```python
from build123d import *

# Parameters (mm, degrees)
SKETCH1_R           = 150
BOSS_EXTRUDE1_DEPTH = 10
SKETCH2_R           = 2
CUT_EXTRUDE1_DEPTH  = 10


with BuildPart() as part:
    # Sketch1 → Boss-Extrude1 (new body)
    with BuildSketch(Plane(origin=(0, 0, 0), x_dir=(1, 0, 0), z_dir=(0, 1, 0))):
        with Locations(Location((0, 0, 0), (0, 0, 270))):
            Circle(SKETCH1_R)
    extrude(amount=BOSS_EXTRUDE1_DEPTH)

    # Sketch2 → Cut-Extrude1 (cut)
    with BuildSketch(Plane(origin=(0, 10, 0), x_dir=(1, 0, 0), z_dir=(0, 1, 0))):
        with Locations(Location((-14.945, 131.706442493, 0), (0, 0, 270))):
            Circle(SKETCH2_R)
        with Locations(Location((-14.945, 107.646442493, 0), (0, 0, 270))):
            Circle(SKETCH2_R)
        with Locations(Location((14.945, 107.646442493, 0), (0, 0, 90))):
            Circle(SKETCH2_R)
        with Locations(Location((14.945, 131.706442493, 0), (0, 0, 90))):
            Circle(SKETCH2_R)
        with Locations(Location((131.706442493, 14.945, 0), (0, 0, 270))):
            Circle(SKETCH2_R)
        with Locations(Location((131.706442493, -14.945, 0), (0, 0, 90))):
            Circle(SKETCH2_R)
        with Locations(Location((107.646442493, -14.945, 0), (0, 0, 90))):
            Circle(SKETCH2_R)
        with Locations(Location((107.646442493, 14.945, 0), (0, 0, 270))):
            Circle(SKETCH2_R)
        with Locations(Location((14.945, -131.706442493, 0), (0, 0, 270))):
            Circle(SKETCH2_R)
        with Locations(Location((-14.945, -131.706442493, 0), (0, 0, 90))):
            Circle(SKETCH2_R)
        with Locations(Location((-14.945, -107.646442493, 0), (0, 0, 90))):
            Circle(SKETCH2_R)
        with Locations(Location((14.945, -107.646442493, 0), (0, 0, 270))):
            Circle(SKETCH2_R)
        with Locations(Location((-131.706442493, -14.945, 0), (0, 0, 270))):
            Circle(SKETCH2_R)
        with Locations(Location((-131.706442493, 14.945, 0), (0, 0, 90))):
            Circle(SKETCH2_R)
        with Locations(Location((-107.646442493, 14.945, 0), (0, 0, 90))):
            Circle(SKETCH2_R)
        with Locations(Location((-107.646442493, -14.945, 0), (0, 0, 270))):
            Circle(SKETCH2_R)
    extrude(amount=-CUT_EXTRUDE1_DEPTH, mode=Mode.SUBTRACT)


solid = part.part
```
Here's how the part is built. I have some questions about the finished solid (model axes, mm). Coordinates: 2 decimals unless noted, no trailing zeros. Loops run counter-clockwise (first coordinate to the right, second up) from the corner with the lowest first, then second, coordinate; pieces in that order, holes last. Notation, with made-up numbers: M 51,-26.5 L 68,-26.5 A25 ccw 68,-2.5 Z; hole C 72.5,-17.5 d3. An arc over 180 degrees is marked long. One line per item, written item: value.
1. Imagine slicing it at C-C (z = 50.5). List the corners of the cut face in (x, y) for me.
Geometry says:
outline: M -141.24,0 L 141.24,0 L 141.24,10 L -141.24,10 Z
2. Imagine slicing it at A-A (y = 2). State how many separate pieces and enclosed holes the cut face has, and give its area (3 significant figures).
Geometry says:
separate pieces: 1
enclosed holes: 16
area: 70,500 mm2
3. Please list where these lines run through material, in increasing order: probe 1 along Z at (x, y) = (106.5, 5); probe 2 along Z at (x, y) = (16.5, 9); probe 3 along X at (y, z) = (9.25, -132.5).
Geometry says:
probe 1: z = -105.63 to -16.58, -13.31 to 13.31, 16.58 to 105.63
probe 2: z = -149.09 to -132.96, -130.45 to -108.9, -106.39 to 106.39, 108.9 to 130.45, 132.96 to 149.09
probe 3: x = -70.31 to -16.78, -13.11 to 13.11, 16.78 to 70.31
4. Imagine slicing it at B-B (x = -31.5). List the corners of the cut face in (y, z) for me, and give its area (3 significant figures).
Geometry says:
outline: M 0,-146.66 L 10,-146.66 L 10,146.66 L 0,146.66 Z
area: 2,930 mm2
5. Will these pins go through, and if not, where does the flat tip stop? pin 1 Ø1 at (y, z) = (5.5, 102.5) entering from +X; pin 2 Ø3 at (y, z) = (2, -66) entering from +X; pin 3 Ø1 at (x, y) = (108.5, 1.5) entering from +Z.
Geometry says:
pin 1: stops at x = 109.98
pin 2: stops at x = 135.42
pin 3: stops at z = 104.1
